Build history of the part. All positions in model axes, mm. Give positions to 0.01 mm unless a question says otherwise; leave off trailing zeros. Order: outer loops, then holes, each group sorted by start corner. A loop starts at its lowest first (then second) coordinate and runs counter-clockwise, first axis right, second up. Notation, with made-up numbers: (-15.5, 75) - (32.5, 75) arc R22 ccw to (32.5, 87) - close; hole circle Ø9 at (67.5, 11.5). An arc over 180 degrees is marked (long way). Write each question's results on one line, items separated by ' | '. Start each with the question number.
from build123d import *

# Parameters (mm, degrees)
SKETCH3_R          = 11
SKETCH3_R_2        = 10.2
CUT_EXTRUDE1_REACH = 197.895
SKETCH4_R          = 3.3
SKETCH5_R          = 3.3
CUT_EXTRUDE2_DEPTH = 196.894862351
SKETCH6_W          = 5.2
SKETCH6_H          = 5.111091306
CUT_EXTRUDE3_DEPTH = 196.894862351


with BuildPart() as part:
    # Sweep2: sweep along a path in Sketch1
    with BuildLine(Plane.XY) as sweep2_path:
        Line((108.839588828, 0), (92.239588828, 0))
        Line((92.239588828, 0), (-92.239588828, 0))
        ThreePointArc((-92.239588828, 0), (-124.360019313, -10.591729527), (-143.88004565, -38.211927945))
        Line((-143.88004565, -38.211927945), (-154.760411172, -73.8))
        Line((-154.760411172, -73.8), (-160.324709574, -92))
    # Sketch3 → Sweep2 (sweep)
    with BuildSketch(Plane(origin=(92.239588828, 0, 0), x_dir=(0, 0, -1), z_dir=(1, 0, 0))):
        Circle(SKETCH3_R)
        Circle(SKETCH3_R_2, mode=Mode.SUBTRACT)
    sweep(path=sweep2_path.line)

    # Sketch4 → Cut-Extrude1 (cut, up to next)
    with BuildSketch(Plane.XY, mode=Mode.PRIVATE) as cut_extrude1_sk1:
        with Locations(Location((-154.760411172, -73.8, 0), (0, 0, 163))):
            Circle(SKETCH4_R)
    cut_extrude1_tool1 = extrude(cut_extrude1_sk1.sketch, amount=CUT_EXTRUDE1_REACH, mode=Mode.PRIVATE) & part.part
    # Sketch4 → Cut-Extrude1 (cut, up to next)
    with BuildSketch(Plane.XY, mode=Mode.PRIVATE) as cut_extrude1_sk2:
        Polygon((108.839588828, 2.555545653), (108.839588828, -2.555545653), (105.639588828, -2.555545653), (103.639588828, -2.555545653), (103.639588828, -0.555545653), (103.639588828, 0.555545653), (103.639588828, 2.555545653), (105.639588828, 2.555545653), align=None)
    cut_extrude1_tool2 = extrude(cut_extrude1_sk2.sketch, amount=CUT_EXTRUDE1_REACH, mode=Mode.PRIVATE) & part.part
    # Sketch4 → Cut-Extrude1 (cut, up to next)
    with BuildSketch(Plane.XY, mode=Mode.PRIVATE) as cut_extrude1_sk3:
        with BuildLine():
            Line((91.989588828, -5.5), (92.489588828, -5.5))
            ThreePointArc((92.489588828, -5.5), (95.141239258, -4.401650429), (96.239588828, -1.75))
            Line((96.239588828, -1.75), (96.239588828, 1.75))
            ThreePointArc((96.239588828, 1.75), (95.141239258, 4.401650429), (92.489588828, 5.5))
            Line((92.489588828, 5.5), (91.989588828, 5.5))
            ThreePointArc((91.989588828, 5.5), (89.337938399, 4.401650429), (88.239588828, 1.75))
            Line((88.239588828, 1.75), (88.239588828, -1.75))
            ThreePointArc((88.239588828, -1.75), (89.337938399, -4.401650429), (91.989588828, -5.5))
        make_face()
    cut_extrude1_tool3 = extrude(cut_extrude1_sk3.sketch, amount=CUT_EXTRUDE1_REACH, mode=Mode.PRIVATE) & part.part
    add(cut_extrude1_tool1.solids().sort_by_distance((-154.760411, -73.8, 0))[0], mode=Mode.SUBTRACT)
    add(cut_extrude1_tool2.solids().sort_by_distance((106.239589, 0, 0))[0], mode=Mode.SUBTRACT)
    add(cut_extrude1_tool3.solids().sort_by_distance((92.239589, 0, 0))[0], mode=Mode.SUBTRACT)

    # Sketch5 → Cut-Extrude2 (cut, through all)
    with BuildSketch(Plane.XY):
        with Locations(Location((-154.760411172, -73.8, 0), (0, 0, 163))):
            Circle(SKETCH5_R)
    extrude(amount=-CUT_EXTRUDE2_DEPTH, mode=Mode.SUBTRACT)

    # Sketch6 → Cut-Extrude3 (cut, through all)
    with BuildSketch(Plane.XY):
        with Locations((106.239588828, 0)):
            Rectangle(SKETCH6_W, SKETCH6_H)
    extrude(amount=-CUT_EXTRUDE3_DEPTH, mode=Mode.SUBTRACT)


solid = part.part
Item 1: Flat gauge pins, fed straight in: pin 1 Ø4 at (x, z) = (-17.5, 8.5) entering from +Y; pin 2 Ø5.5 at (x, y) = (-154.76, -73.8) entering from +Z; pin 3 Ø1 at (x, z) = (-17.5, 3) entering from +Y; pin 4 Ø0.9 at (x, z) = (106.5, 10.5) entering from -Y. Where does each tip first touch, or does it go through?
Item 2: Cut at A-A, the plane z = -3. List the corners of the cut face in (x, y), then the cut area to 3 significant figures.
Item 3: Cut at B-B, the plane x = 41. List the corners of the cut face in (y, z).
Item 4: Probe line 1 along Y through (x, z) = (-6, 0.75); line 2 along Y through (x, z) = (94.5, -6.75); line 3 along X through (y, z) = (-43.5, 0.25). List the from-to ranges inside material, lowest first. Write a range as from..to.
Item 5: Two-plate mould, pull along Z, no slides. Class faces 1 (the cylindrical face through (6.892, 9.049, -4.707)), 2 (the flat face through (108.84, -10.6, 0)), 3 (the cylindrical face through (6.89, 10.74, 2.38)): +Z half, -Z half, draft (parallel to the pull), parting line (faces both ways), or undercut.
Values found:
1) pin 1: stops at y = 8.87 | pin 2: passes through | pin 3: stops at y = 10.71 | pin 4: stops at y = -4.47
2) outline: (-170.45, -88.91) - (-169.65, -89.15) - (-153.2, -35.36) arc R63.75 cw to (-92.24, 9.75) - (108.84, 9.75) - (108.84, 10.58) - (-92.24, 10.58) arc R64.58 ccw to (-154, -35.12) - close; (-151, -94.85) - (-150.2, -95.09) - (-133.76, -41.31) arc R43.42 cw to (-92.24, -10.58) - (108.84, -10.58) - (108.84, -9.75) - (-92.24, -9.75) arc R44.25 ccw to (-134.56, -41.06) - close | area: 544 mm2
3) outline: circle Ø22 at (0, 0); hole circle Ø20.4 at (0, 0)
4) line 1: y = -10.97..-10.17, 10.17..10.97 | line 2: y = -8.69..-7.65, 7.65..8.69 | line 3: x = -157..-156.16, -134.83..-134
5) face 1: undercut | face 2: draft | face 3: parting line
